Part model, mm, in its own coordinate system. Round coordinates to 2 decimals unless told otherwise and drop trailing zeros. Write each loop counter-clockwise with the first axis right and the second up, starting at its lowest first coordinate (ties: lowest second). Pieces come first, ordered by that corner, then holes. Notation, with made-up numbers: M 31.25,74.5 L 52.25,74.5 A7 ccw 52.25,87.5 Z; hole C 56.5,-9 d5. An arc over 180 degrees is marked long. Use one line per item in the form item = value. Start each with the question number.
Item 1: Cut at C-C, the plane z = -0.55. Give the cut face in (x, y), then the cut area to 3 significant figures.
Item 2: Cut at A-A, the plane x = 0. Give the cut face in (y, z).
Item 3: Probe L1, parallel to Y at x = 0, z = 0.7; L2, parallel to Y at x = -1, z = -1.1. List the from-to ranges inside material, lowest first.
Item 4: Cut at B-B, the plane x = -6.5. Give the cut face in (y, z), then the cut area to 3 significant figures.
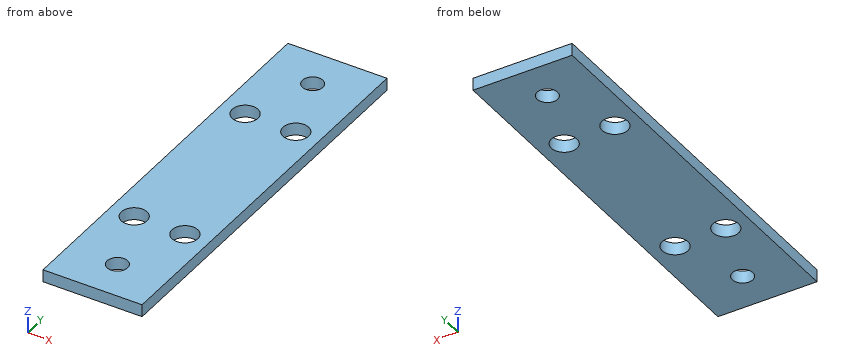
from build123d import *

# Parameters (mm, degrees)
F0_W     = 25.4
F0_H     = 3.175
F1_DEPTH = 101.6
F2_R     = 2.6162
F2_R_2   = 3.302
F3_DEPTH = 3.176


with BuildPart() as f1:
    # F0 (on Front) → F1 (new body)
    with BuildSketch(Plane.XZ):
        Rectangle(F0_W, F0_H)
    extrude(amount=F1_DEPTH)

    # F2 (on face) → F3 (cut, through all)
    with BuildSketch(Plane.XY.offset(1.5875)):
        with Locations((0, -91.2876)):
            Circle(F2_R)
        with Locations((0, -10.3124)):
            Circle(F2_R)
        with Locations((-6.5024, -27.8003)):
            Circle(F2_R_2)
        with Locations((6.5024, -27.8003)):
            Circle(F2_R_2)
        with Locations((6.5024, -73.7997)):
            Circle(F2_R_2)
        with Locations((-6.5024, -73.7997)):
            Circle(F2_R_2)
    extrude(amount=-F3_DEPTH, mode=Mode.SUBTRACT)


solid = f1.part
Model answer:
q1.outline = M -12.7,-101.6 L 12.7,-101.6 L 12.7,0 L -12.7,0 Z; hole C -6.5,-73.8 d6.6; hole C -6.5,-27.8 d6.6; hole C 0,-91.29 d5.23; hole C 0,-10.31 d5.23; hole C 6.5,-73.8 d6.6; hole C 6.5,-27.8 d6.6
q1.area = 2,400 mm²
q2.outline = M -101.6,-1.59 L -93.9,-1.59 L -93.9,1.59 L -101.6,1.59 Z; M -88.67,-1.59 L -12.93,-1.59 L -12.93,1.59 L -88.67,1.59 Z; M -7.7,-1.59 L 0,-1.59 L 0,1.59 L -7.7,1.59 Z
q3.L1 = -101.6 to -93.9, -88.67 to -12.93, -7.7 to 0
q3.L2 = -101.6 to -93.71, -88.87 to -12.73, -7.89 to 0
q4.outline = M -101.6,-1.59 L -77.1,-1.59 L -77.1,1.59 L -101.6,1.59 Z; M -70.5,-1.59 L -31.1,-1.59 L -31.1,1.59 L -70.5,1.59 Z; M -24.5,-1.59 L 0,-1.59 L 0,1.59 L -24.5,1.59 Z
q4.area = 281 mm²
